```python
from build123d import *

# Parameters (mm, degrees)
F1_DEPTH = 31.75
F2_W     = 19.05
F2_H     = 19.05
F3_DEPTH = 19.05
F5_DEPTH = 19.05
F7_DEPTH = 19.05


# Not quite as in the source:
# - a length typed as a fraction of an inch, garbled in the dataset ("3 / 203.2 mm" for 3/8 in), is restored


with BuildPart() as f1:
    # F0 (on Front) → F1 (new body)
    with BuildSketch(Plane.XZ):
        Polygon((-50.8, 0), (0, 0), (0, 31.75), (-38.1, 31.75), (-50.8, 12.7), align=None)
    extrude(amount=F1_DEPTH)

    # F2 (on Front) → F3 (cut)
    with BuildSketch(Plane.XZ):
        with Locations((-9.525, 22.225)):
            Rectangle(F2_W, F2_H)
    extrude(amount=F3_DEPTH, mode=Mode.SUBTRACT)

    # F4 (on Front) → F5 (cut)
    with BuildSketch(Plane.XZ):
        Polygon((-31.6195416782, 13.0910674021), (-31.3020864666, 32.1384221315), (-37.6520864666, 32.1384221315), (-50.6695416782, 13.0910674021), align=None)
    extrude(amount=F5_DEPTH, mode=Mode.SUBTRACT)

    # F6 (on Front) → F7 (cut)
    with BuildSketch(Plane.XZ):
        Polygon((-34.3563221395, 12.8449322656), (-34.3563221395, 35.7176738393), (-68.0936202407, 12.8449322656), align=None)
    extrude(amount=F7_DEPTH, mode=Mode.SUBTRACT)


solid = f1.part
```
Geometry check sheet. Reference: the model listing, model coordinates, mm. A direction names the side the tool comes from. Coordinates: 2 decimals unless noted, no trailing zeros. Write each loop counter-clockwise with the first axis right and the second up, starting at its lowest first coordinate (ties: lowest second). Pieces come first, ordered by that corner, then holes. Notation, with made-up numbers: M 68.25,11.5 L 101.25,11.5 A14 cw 101.25,16.5 Z; hole C 89,60.25 d2. An arc over 180 degrees is marked long. One line per item, written item: value. Start each with the question number.
(1) Scan lines: line 1 along Z through (x, y) = (-14.5, -18); line 2 along Y through (x, z) = (-7, 25); line 3 along Z through (x, y) = (-45, -16). Record each from-to range of solid material in increasing order. Write a range as [from, to].
(2) Sectioned sample at B-B, the plane y = -8. Enter the section's corners in (x, z), and give its area (3 significant figures).
(3) Tool access check on faces 1 (the face through (-10, -19.05, 22)), 2 (the face through (0, -19, 12)), 3 (the face through (-43, -9, 12.845)). Record the directions out of +Z, -Z, +X, -X, +Y, -Y that give a thin tool (end or side, any length) a straight path to the whole face; none if there is none.
(4) Depth check by flat-ended pin: pin 1 (2 mm diameter, centred on y = -15.5, z = 24.5, fed in from +X); pin 2 (5 mm diameter, centred on y = -15.5, z = 6.5, fed in from +X); pin 3 (13 mm diameter, centred on x = -39, y = -5.5, fed in from +Z); pin 4 (15 mm diameter, centred on x = -5, z = 22.5, fed in from +Y). Enter the tip coordinate at first touch or a pass-through.
(5) Sectioned sample at D-D, the plane x = -4.5. Enter the section's corners in (y, z).
(6) Sectioned sample at C-C, the plane z = 15. Enter the section's corners in (x, y).
(7) Sectioned sample at A-A, the plane x = -33.5. Enter the section's corners in (y, z).
Filled sheet:
1. line 1: [0, 12.7]
1. line 2: [-31.75, -19.05]
1. line 3: [0, 12.84]
2. outline: M -50.8,0 L 0,0 L 0,12.7 L -19.05,12.7 L -19.05,31.75 L -31.31,31.75 L -31.62,13.09 L -34.36,13.09 L -34.36,12.84 L -50.7,12.84 L -50.8,12.7 Z
2. area: 885 mm²
3. face 1: +Z, +X, +Y
3. face 2: +Z, -Z, +X, +Y, -Y
3. face 3: +Z, -X, +Y
4. pin 1: x = -19.05
4. pin 2: x = 0
4. pin 3: z = 13.09
4. pin 4: y = -19.05
5. outline: M -31.75,0 L 0,0 L 0,12.7 L -19.05,12.7 L -19.05,31.75 L -31.75,31.75 Z
6. outline: M -49.27,-31.75 L 0,-31.75 L 0,-19.05 L -19.05,-19.05 L -19.05,0 L -31.59,0 L -31.59,-19.05 L -49.27,-19.05 Z
7. outline: M -31.75,0 L 0,0 L 0,13.09 L -19.05,13.09 L -19.05,31.75 L -31.75,31.75 Z
